Here's how the part is built. I have some questions about the finished solid (model axes, mm). A direction names the side the tool comes from. Coordinates: 2 decimals unless noted, no trailing zeros. Loops run counter-clockwise (first coordinate to the right, second up) from the corner with the lowest first, then second, coordinate; pieces in that order, holes last. Notation, with made-up numbers: M 60,14 L 86,14 A21 ccw 86,49 Z; hole C -28,69.5 d1. An arc over 180 degrees is marked long. Use one line per item in the form item = value. Start each with the question number.
(1) Imagine slicing it at B-B, the plane x = 119.5. Please give me the cut outline in (y, z).
(2) Imagine slicing it at A-A, the plane z = 0. Please give me the cut outline in (x, y).
(3) On a 3-axis mill with a long thin cutter (end or side, diameter ignored), from which of +Z, -Z, +X, -X, +Y, -Y can I reach the whole of each face in a straight line? I mean faces 1 (the flat face through (290, 6, 0)), 2 (the flat face through (10, 6, 0)), 3 (the conical face through (299.865, -9.631, 0.299)). Say none if no direction works.
(4) Please list where these lines run through material, in increasing order: L1, parallel to X at y = 6.5, z = 5.5; L2, parallel to Y at x = 270.5, z = -3.25; L3, parallel to Z at x = 31, y = -0.5.
(5) Will these pins go through, and if not, where does the flat tip stop? P1, Ø4.5, axis at y = 8.5, z = 4, coming from the -X side; P2, Ø8, axis at x = 7, z = -0.5, coming from the +Y side; P3, Ø5, axis at x = 201.5, y = -6, coming from the -Z side.
```python
from build123d import *

# Parameters (mm, degrees)
SKETCH1_W               = 300
SKETCH1_H               = 10
CUT_EXTRUDE1_DEPTH      = 301.333148354
CUT_EXTRUDE1_DEPTH_BACK = 301.333148354
SKETCH2_W               = 20
SKETCH2_H               = 4
CHAMFER1_SIZE           = 0.5


with BuildPart() as part:
    # Sketch1 → Revolve1 (revolve)
    with BuildSketch(Plane.XY, mode=Mode.PRIVATE) as revolve1_sk:
        with Locations((150, 5)):
            Rectangle(SKETCH1_W, SKETCH1_H)
    revolve(revolve1_sk.sketch.rotate(Axis((0, 0, 0), (1, 0, 0)), 90), axis=Axis((0, 0, 0), (1, 0, 0)))

    # Sketch2 → Cut-Extrude1 (cut, two sides: drawn at the far end of the back side and taken through both)
    with BuildSketch(Plane.XY.offset(-CUT_EXTRUDE1_DEPTH_BACK)):
        with Locations((10, 8)):
            Rectangle(SKETCH2_W, SKETCH2_H)
        with Locations((290, 8)):
            Rectangle(SKETCH2_W, SKETCH2_H)
    extrude(amount=CUT_EXTRUDE1_DEPTH + CUT_EXTRUDE1_DEPTH_BACK, mode=Mode.SUBTRACT)

    # Chamfer1
    chamfer1_edges = [part.edges().sort_by_distance(p)[0] for p in [
        (0, 6, 0),
        (300, -9.486832981, -3.16227766),
        (300, 6, 0),
        (0, -9.486832981, -3.16227766),
    ]]
    chamfer(chamfer1_edges, length=CHAMFER1_SIZE)


solid = part.part
```
Answer:
q1.outline = C 0,0 d20
q2.outline = M 0,-9.5 L 0.5,-10 L 299.5,-10 L 300,-9.5 L 300,5.5 L 299.5,6 L 280,6 L 280,10 L 20,10 L 20,6 L 0.5,6 L 0,5.5 Z
q3.face_1 = +Z, -Z, +X, +Y
q3.face_2 = +Z, -Z, -X, +Y
q3.face_3 = +X
q4.L1 = 20 to 280
q4.L2 = -9.46 to 9.46
q4.L3 = -9.99 to 9.99
q5.P1 = 20
q5.P2 = 6
q5.P3 = -9.37
